Check sheet for the modelled part. Datum: model origin and axes. Units: mm. Give positions to 0.01 mm unless a question says otherwise; leave off trailing zeros. Order: outer loops, then holes, each group sorted by start corner. A loop starts at its lowest first (then second) coordinate and runs counter-clockwise, first axis right, second up.
```python
from build123d import *

# Parameters (mm, degrees)
F0_W     = 104
F0_H     = 75
F1_DEPTH = 5
F2_R     = 5
F4_D     = 2.75
F5_R     = 1
F6_R     = 1


with BuildPart() as f1:
    # F0 (on Front) → F1 (new body)
    with BuildSketch(Plane.XZ):
        Rectangle(F0_W, F0_H)
    extrude(amount=-F1_DEPTH)

    # F2
    f2_edges = [f1.edges().sort_by_distance(p)[0] for p in [
        (-52, 2.5, 37.5),
        (52, 2.5, 37.5),
        (52, 2.5, -37.5),
        (-52, 2.5, -37.5),
    ]]
    fillet(f2_edges, radius=F2_R)

    # F4 (through all)
    with Locations(Plane.XZ):
        with Locations((-39, 24.5), (19, 24.5), (19, -24.5), (-39, -24.5)):
            Hole(F4_D / 2)

    # F5
    f5_edges = [f1.edges().sort_by_distance(p)[0] for p in [
        (-52, 5, 0),
    ]]
    fillet(f5_edges, radius=F5_R)

    # F6
    f6_edges = [f1.edges().sort_by_distance(p)[0] for p in [
        (0, 0, 37.5),
    ]]
    fillet(f6_edges, radius=F6_R)


solid = f1.part
```
(1) Release check for a two-part mould opening along Z. For faces 1 (the face through (-1, 0, 1)), 2 (the face through (20.013, 2.535, -23.571)), 3 (the face through (-1, 2, -37.5)) record: released by +Z, released by -Z, zero draft, split by the parting line, or undercut.
Response values:
face 1: zero draft
face 2: undercut
face 3: released by -Z
(2) Cross-section at A-A on x = -39. Enter the section's corners in (y, z) (3 decimals), then the cut area to 3 significant figures.
Response values:
outline: (0, -36.5) arc R1 ccw to (1, -37.5) - (4, -37.5) arc R1 ccw to (5, -36.5) - (5, -25.875) - (0, -25.875) - close; (0, -23.125) - (5, -23.125) - (5, 23.125) - (0, 23.125) - close; (0, 25.875) - (5, 25.875) - (5, 36.5) arc R1 ccw to (4, 37.5) - (1, 37.5) arc R1 ccw to (0, 36.5) - close
area: 347 mm2
(3) Material ranges on L1, parallel to Z at x = 19, y = 3.9 (3 decimals); L2, parallel to X at y = 4.2, z = 25; L3, parallel to X at y = 4.1, z = 5, recorded low to high.
Response values:
L1: z = -37.5 to -25.875, -23.125 to 23.125, 25.875 to 37.5
L2: x = -51.98 to -40.28, -37.72 to 17.72, 20.28 to 51.98
L3: x = -51.99 to 51.99
(4) Cross-section at B-B on z = -24.5. Enter the section's corners in (x, y) (3 decimals).
Response values:
outline: (-52, 1) arc R1 ccw to (-51, 0) - (-40.375, 0) - (-40.375, 5) - (-51, 5) arc R1 ccw to (-52, 4) - close; (-37.625, 0) - (17.625, 0) - (17.625, 5) - (-37.625, 5) - close; (20.375, 0) - (51, 0) arc R1 ccw to (52, 1) - (52, 4) arc R1 ccw to (51, 5) - (20.375, 5) - close
